Geometry: final body of the model. Coordinates: model frame, mm. A direction names the side the tool comes from. Give positions to 0.01 mm unless a question says otherwise; leave off trailing zeros. Write each loop counter-clockwise with the first axis right and the second up, starting at its lowest first coordinate (ties: lowest second). Pieces come first, ordered by that corner, then holes. Notation, with made-up numbers: (20.5, 63) -> (47.5, 63) arc R8 ccw to (47.5, 72) -> close; hole circle Ø3 at (81.25, 87.5). An arc over 180 degrees is marked (long way). Answer in a Markdown table with one row per item. Add a question column.
Item 1: Access query for faces 1 (the flat face through (-4.6, 7.5, -2)), 2 (the cylindrical face through (9.376, 3.888, -1.507)), 3 (the cylindrical face through (-1.545, 6.956, -91.358)). Directions: +Z, -Z, +X, -X, +Y, -Y. A direction counts if a zero-diameter tool reaches every point of the face in a straight line with its end or side. Return the directions, or none.
Item 2: Section query B-B on z = -72. Output: boundary loops of the cut face in (x, y), plus the area to 3 significant figures.
Item 3: Material intervals for probe 1 along Y at (x, z) = (-1.25, -52.5); probe 2 along Y at (x, z) = (0, -31); probe 3 along X at (y, z) = (-2, -11.5), sorted ascending. Write a range as from..to.
Item 4: Section query A-A on z = -90.5. Output: boundary loops of the cut face in (x, y) (3 decimals).
Item 5: Draft query along Z for faces 4 (the flat face through (2, 6, -99.5)), 5 (the cylindrical face through (5.77, -1.82, -49.56)), 6 (the conical face through (4, 8, -5)). Return one class per face: +Z half, -Z half, draft (parallel to the pull), parting line (faces both ways), or undercut.
Item 6: First-contact query: P1, Ø11, axis at x = 0, y = 0, coming from the -Z side; P2, Ø1, axis at x = -0.5, z = -43.5, coming from the -Y side; P3, Ø10, axis at x = 7, z = -36, coming from the +Y side; P4, Ø2, axis at y = -4.5, z = -34.5, coming from the -X side. Flat tips, straight axial feed; report the tip coordinate or a pass-through.
```python
from build123d import *

# Parameters (mm, degrees)
CHAMFER_1_SIZE2 = 1.6
CHAMFER_1_SIZE  = 2
FILLET_1_R      = 1
CHAMFER_2_SIZE  = 0.5
CHAMFER_3_SIZE  = 1


with BuildPart() as part:
    # 스케치2 → 회전1 (revolve)
    with BuildSketch(Plane(origin=(0, 0, 0), x_dir=(0, 0, -1), z_dir=(1, 0, 0)), mode=Mode.PRIVATE) as revolve_1_sk:
        Polygon((76, -9), (83.5, -7.125), (99.5, -7.125), (99.5, -6.05), (83.5, -6.05), (0, -6.05), (0, -10.15), (2, -10.15), (2, -8.55), (4.5, -8.55), (4.5, -10.15), align=None)
    revolve(revolve_1_sk.sketch.rotate(Axis((0, 0, 0), (0, 0, -1)), 270), axis=Axis((0, 0, 0), (0, 0, -1)))

    # 모따기1
    chamfer_1_edges = [part.edges().sort_by_distance(p)[0] for p in [
        (-10.15, 0, -4.5),
    ]]
    chamfer_1_side = [part.faces().sort_by_distance(p)[0] for p in [
        (-10.149485381, 0, -4.531995862),
    ]]
    chamfer(chamfer_1_edges, length=CHAMFER_1_SIZE - 0.0001, length2=CHAMFER_1_SIZE2 - 0.0001, reference=chamfer_1_side[0])  # a hair under: the kernel refuses the full size

    # 필렛1
    fillet_1_edges = [part.edges().sort_by_distance(p)[0] for p in [
        (-10.15, 0, 0),
    ]]
    fillet(fillet_1_edges, radius=FILLET_1_R)

    # 모따기2
    chamfer_2_edges = [part.edges().sort_by_distance(p)[0] for p in [
        (-7.125, 0, -99.5),
    ]]
    chamfer(chamfer_2_edges, length=CHAMFER_2_SIZE)

    # 모따기3
    chamfer_3_edges = [part.edges().sort_by_distance(p)[0] for p in [
        (-6.05, 0, 0),
    ]]
    chamfer(chamfer_3_edges, length=CHAMFER_3_SIZE)


solid = part.part
```
Findings below:
| question | item | result |
|---|---|---|
| 1 | face 1 | none |
| 1 | face 2 | +Z, -Z |
| 1 | face 3 | -Z |
| 2 | outline | circle Ø18.13 at (0, 0); hole circle Ø12.1 at (0, 0) |
| 2 | area | 143 mm^2 |
| 3 | probe 1 | y = -9.29..-5.92, 5.92..9.29 |
| 3 | probe 2 | y = -9.72..-6.05, 6.05..9.72 |
| 3 | probe 3 | x = -9.84..-5.71, 5.71..9.84 |
| 4 | outline | circle Ø14.25 at (0, 0); hole circle Ø12.1 at (0, 0) |
| 5 | face 4 | -Z half |
| 5 | face 5 | draft |
| 5 | face 6 | undercut |
| 6 | P1 | passes through |
| 6 | P2 | stops at y = -9.53 |
| 6 | P3 | stops at y = 9.44 |
| 6 | P4 | stops at x = -9.01 |
